from build123d import *

# Parameters (mm, degrees)
SKETCH_1_R          = 1.5
SKETCH_1_R_2        = 7.02
SKETCH_1_W          = 4.3
SKETCH_1_H          = 8.3
EXTRUDE_1_DEPTH     = 4
CUT_EXTRUDE_1_DEPTH = 4
SKETCH_3_R          = 2
CUT_EXTRUDE_2_DEPTH = 4
SKETCH_4_W          = 10
SKETCH_4_H          = 47.093490756
EXTRUDE_2_DEPTH     = 4
SKETCH_7_R          = 2
CUT_EXTRUDE_3_DEPTH = 4
FILLET_1_R          = 2


with BuildPart() as part:
    # 草图1 → 凸台-拉伸1 (new body)
    with BuildSketch(Plane.XY):
        with BuildLine():
            Line((230.542857143, -31.145714286), (199.556073527, -38.70591431))
            Line((199.556073527, -38.70591431), (174.542857143, -46.295714286))
            Line((174.542857143, -46.295714286), (34.542857143, -46.295714286))
            Line((34.542857143, -46.295714286), (2.692857143, -38.295714286))
            Line((2.692857143, -38.295714286), (-5.457142857, -38.295714286))
            Line((-5.457142857, -38.295714286), (-5.457142857, 41.704285714))
            Line((-5.457142857, 41.704285714), (9.542857143, 41.704285714))
            Line((9.542857143, 41.704285714), (9.542857143, 14.854285714))
            Line((9.542857143, 14.854285714), (18.542857143, 14.854285714))
            Line((18.542857143, 14.854285714), (18.542857143, 41.704285714))
            Line((18.542857143, 41.704285714), (199.542857143, 41.704285714))
            Line((199.542857143, 41.704285714), (230.542857143, 30.854285714))
            ThreePointArc((230.542857143, 30.854285714), (261.542857143, -0.145714286), (230.542857143, -31.145714286))
        make_face()
        with Locations((0.542857143, 29.854285714)):
            Circle(SKETCH_1_R, mode=Mode.SUBTRACT)
        with Locations((0.542857143, -0.145714286)):
            Circle(SKETCH_1_R, mode=Mode.SUBTRACT)
        with Locations((0.542857143, -30.145714286)):
            Circle(SKETCH_1_R, mode=Mode.SUBTRACT)
        with Locations((230.542857143, -0.145714286)):
            Circle(SKETCH_1_R_2, mode=Mode.SUBTRACT)
        with Locations((0.542857143, 14.854285714)):
            Rectangle(SKETCH_1_W, SKETCH_1_H, mode=Mode.SUBTRACT)
        with Locations((0.542857143, -15.145714286)):
            Rectangle(SKETCH_1_W, SKETCH_1_H, mode=Mode.SUBTRACT)
    extrude(amount=EXTRUDE_1_DEPTH)

    # 草图2 → 切除-拉伸1 (cut)
    with BuildSketch(Plane.XY.offset(4)):
        with BuildLine():
            Line((59.099206329, 22.4106349), (50.542857143, 30.966984086))
            Line((50.542857143, 30.966984086), (19.430158771, -0.145714286))
            Line((19.430158771, -0.145714286), (50.542857143, -31.258412658))
            Line((50.542857143, -31.258412658), (81.655555515, -0.145714286))
            Line((81.655555515, -0.145714286), (73.099206329, 8.4106349))
            ThreePointArc((73.099206329, 8.4106349), (74.584487703, 23.895916275), (59.099206329, 22.4106349))
        make_face()
    extrude(amount=-CUT_EXTRUDE_1_DEPTH, mode=Mode.SUBTRACT)

    # 草图3 → 切除-拉伸2 (cut)
    with BuildSketch(Plane.XY.offset(4)):
        with Locations((27.542857143, 35.704285714)):
            Circle(SKETCH_3_R)
        with Locations((112.542857143, 35.704285714)):
            Circle(SKETCH_3_R)
        with Locations((197.542857143, 35.704285714)):
            Circle(SKETCH_3_R)
        with Locations((112.542857143, -34.295714286)):
            Circle(SKETCH_3_R)
        with Locations((197.542857143, -34.295714286)):
            Circle(SKETCH_3_R)
        with Locations((27.542857143, -34.295714286)):
            Circle(SKETCH_3_R)
        Polygon((187.542857143, -24.295714286), (140.41622539, -24.295714286), (187.542857143, 14.51445304), align=None)
        Polygon((122.542857143, 25.704285714), (169.669488896, 25.704285714), (122.542857143, -13.105881612), align=None)
    extrude(amount=-CUT_EXTRUDE_2_DEPTH, mode=Mode.SUBTRACT)

    # 草图4 → 凸台-拉伸2 (add)
    with BuildSketch(Plane.XY.offset(4)):
        with Locations((139.542857143, 15.704285714)):
            Rectangle(SKETCH_4_W, SKETCH_4_H)
    extrude(amount=-EXTRUDE_2_DEPTH)

    # 草图7 → 切除-拉伸3 (cut)
    with BuildSketch(Plane.XY.offset(4)):
        with Locations((190.542857143, -0.145714286)):
            Circle(SKETCH_7_R)
        with Locations((140.542857143, 16.354285714)):
            Circle(SKETCH_7_R)
        with Locations(Location((140.542857143, -16.645714286, 0), (0, 0, 180))):
            Circle(SKETCH_7_R)
        Polygon((10.655357143, -40.295714286), (194.316671838, -40.295714286), (206.19710926, -67.618852766), (10.655357143, -65.874099546), align=None)
    extrude(amount=-CUT_EXTRUDE_3_DEPTH, mode=Mode.SUBTRACT)

    # 圆角1
    fillet_1_edges = [part.edges().sort_by_distance(p)[0] for p in [
        (187.542857143, 14.51445304, 2),
        (187.542857143, -24.295714286, 2),
        (140.41622539, -24.295714286, 2),
        (122.542857143, -13.105881612, 2),
        (122.542857143, 25.704285714, 2),
        (169.669488896, 25.704285714, 2),
        (134.542857143, -3.223528671, 2),
        (144.542857143, 5.011765447, 2),
        (144.542857143, 25.704285714, 2),
        (134.542857143, 25.704285714, 2),
        (9.542857143, 41.704285714, 2),
        (18.542857143, 41.704285714, 2),
    ]]
    fillet(fillet_1_edges, radius=FILLET_1_R)


solid = part.part
CAD build for the part. Positions are in the model's coordinates, mm. A direction names the side the tool comes from. Coordinates: 2 decimals unless noted, no trailing zeros. Order: outer loops, then holes, each group sorted by start corner. A loop starts at its lowest first (then second) coordinate and runs counter-clockwise, first axis right, second up.
Item 1: Drill centre lines: L1, parallel to Y at x = 181.5, z = 2.6; L2, parallel to Y at x = 191, z = 3.8; L3, parallel to X at y = 2.5, z = 2.9. Where is each one in solid material? Low to high.
Check sheet entries:
L1: y = -40.3 to -24.3, 9.54 to 41.7
L2: y = -40.3 to -2.09, 1.8 to 41.7
L3: x = -5.46 to 22.08, 79.01 to 122.54, 134.54 to 172.95, 187.54 to 224.04, 237.05 to 261.43
Item 2: Two-plate mould, pull along X, no slides. Class faces 3 (the face through (130, -8, 4)), 4 (the face through (215.27, -34.87, 1.97)), 5 (the face through (65.9, -15.9, 2)), 6 (the face through (74.758, 23.718, 2.028)): +X half, -X half, draft (parallel to the pull), parting line (faces both ways), or undercut.
Check sheet entries:
face 3: draft
face 4: +X half
face 5: undercut
face 6: undercut
Item 3: 3-axis set-ups, long thin cutter, end or side, ignore diameter. For faces 1 (the face through (261.535, 0.536, 1.972)), 2 (the face through (54.88, 26.63, 2.03)): which of +Z, -Z, +X, -X, +Y, -Y reach the whole face in a straight line?
Check sheet entries:
face 1: +Z, -Z, +X
face 2: +Z, -Z
Item 4: Band-saw the part on B-B on z = 0.95. Give the number of separate pieces and of enclosed holes in the cut face, plus the area to 3 significant figures.
Check sheet entries:
separate pieces: 1
enclosed holes: 19
area: 16,200 mm2
Item 5: Pin check, flat tips, straight feed: pin 1 Ø2.5 at (x, y) = (0.54, -30.15) entering from +Z; pin 2 Ø2 at (y, z) = (5, 2) entering from +X; pin 3 Ø1.2 at (x, z) = (12.5, 2.5) entering from +Y; pin 4 Ø1.2 at (y, z) = (-17, 1) entering from +X. Stop position of each tip, or through.
Check sheet entries:
pin 1: passes through
pin 2: stops at x = 261.26
pin 3: stops at y = 14.85
pin 4: stops at x = 256.94
Item 6: Band-saw the part on A-A on x = 70. List the corners of the cut face in (y, z), plus the area to 3 significant figures.
Check sheet entries:
outline: (-40.3, 0) - (-11.8, 0) - (-11.8, 4) - (-40.3, 4) - close; (26.52, 0) - (41.7, 0) - (41.7, 4) - (26.52, 4) - close
area: 175 mm2
